For this review, use the dimensioned drawing (mm, ordinates from the lowest corner) and the shaded views. A direction names the side the tool comes from. Coordinates: 2 decimals unless noted, no trailing zeros. Loops run counter-clockwise (first coordinate to the right, second up) from the corner with the lowest first, then second, coordinate; pieces in that order, holes last. Notation, with made-up numbers: M -3.5,-21 L 36.5,-21 A25 ccw 36.5,5 Z; hole C 55.5,47.5 d2. An arc over 180 degrees is marked long. Write item = value, one per line.
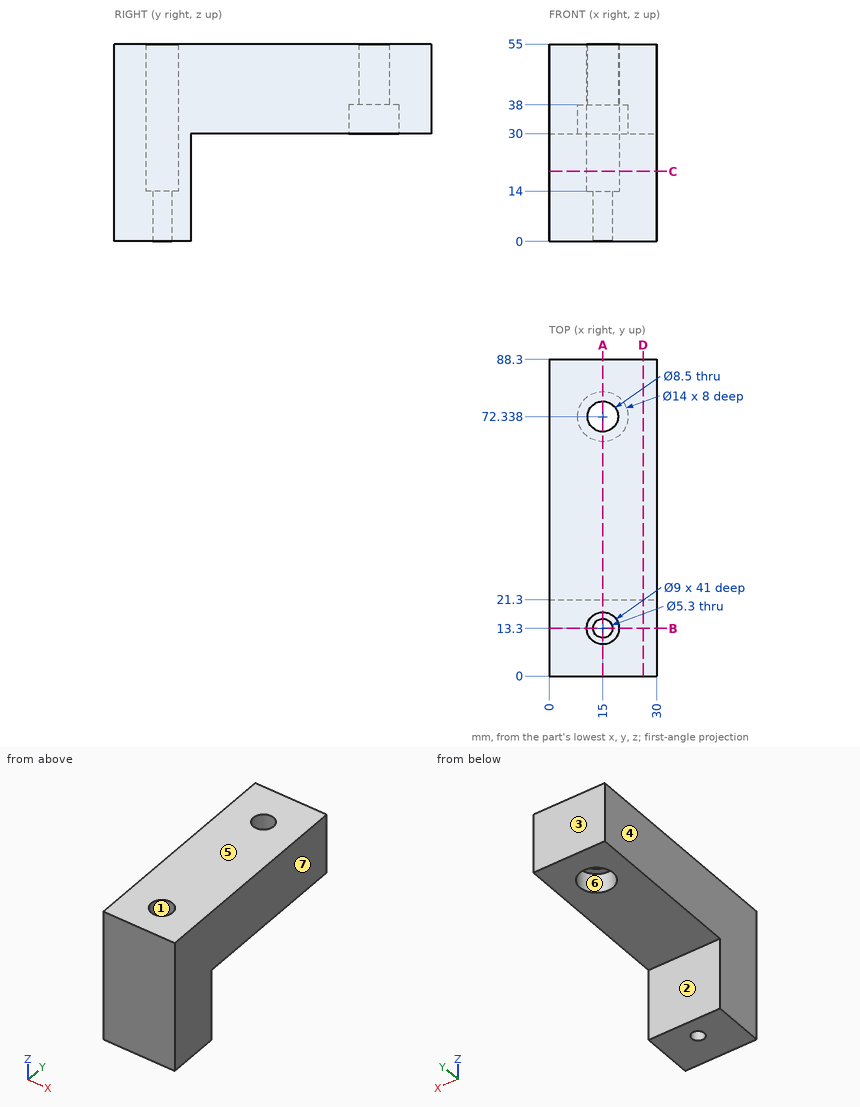
Q1. Draft analysis for pull direction X (two halves, no side actions). For the marked faces 4, 5, 6 and 7, state which applies: +X half, -X half, draft (parallel to the pull), parting line (faces both ways), or undercut.
Solved:
face_4 = -X half
face_5 = draft
face_6 = undercut
face_7 = +X half
Q2. Add section A-A (x = 15). Write out the cut boundary in (y, z), and give its area (3 significant figures).
Solved:
outline = M 0,0 L 10.65,0 L 10.65,14 L 8.8,14 L 8.8,55 L 0,55 Z; M 15.95,0 L 21.3,0 L 21.3,30 L 65.34,30 L 65.34,38 L 68.09,38 L 68.09,55 L 17.8,55 L 17.8,14 L 15.95,14 Z; M 76.59,38 L 79.34,38 L 79.34,30 L 88.3,30 L 88.3,55 L 76.59,55 Z
area = 2,150 mm²
Q3. Add section C-C (z = 19.5). Write out the cut boundary in (x, y), and give its area (3 significant figures).
Solved:
outline = M 0,0 L 30,0 L 30,21.3 L 0,21.3 Z; hole C 15,13.3 d9
area = 575 mm²
Q4. For line 1 along Y through (x, z) = (15, 47.5); line 2 along Y through (x, z) = (15, 34); line 3 along Y through (x, z) = (15, 22.5), list the stretches that pass through material, from the lowest coordinate up.
Solved:
line_1 = 0 to 8.8, 17.8 to 68.09, 76.59 to 88.3
line_2 = 0 to 8.8, 17.8 to 65.34, 79.34 to 88.3
line_3 = 0 to 8.8, 17.8 to 21.3
Q5. Add section B-B (y = 13.3). Write out the cut boundary in (x, z).
Solved:
outline = M 0,0 L 12.35,0 L 12.35,14 L 10.5,14 L 10.5,55 L 0,55 Z; M 17.65,0 L 30,0 L 30,55 L 19.5,55 L 19.5,14 L 17.65,14 Z
Q6. Machinability: for the marked faces 1, 2 and 3, which of the approach directions +Z, -Z, +X, -X, +Y, -Y give a long, thin tool a straight path to every point of the face, cutting with its end or side? Answer none if there is none.
Solved:
face_1 = +Z
face_2 = -Z, +X, -X, +Y
face_3 = +Z, -Z, +X, -X, +Y
Q7. For pin 1 Ø7 at (x, y) = (15, 72.34) entering from -Z; pin 2 Ø4 at (x, z) = (5.5, 17) entering from +Y; pin 3 Ø11 at (x, y) = (16.5, 69) entering from -Z; pin 4 Ø11 at (x, y) = (15, 72.34) entering from -Z, all flat-tipped, find the tip position at first contact; note any pin that passes through.
Solved:
pin_1 = through
pin_2 = 21.3
pin_3 = 30
pin_4 = 38
Q8. Add section D-D (x = 26.25). Write out the cut boundary in (y, z), and give its area (3 significant figures).
Solved:
outline = M 0,0 L 21.3,0 L 21.3,30 L 88.3,30 L 88.3,55 L 0,55 Z
area = 2,850 mm²
